Check sheet for the drawn part. Datum: minimum x, y, z corner. Units: mm. Give positions to 0.01 mm unless a question says otherwise; leave off trailing zeros. Order: outer loops, then holes, each group sorted by start corner. A loop starts at its lowest first (then second) coordinate and runs counter-clockwise, first axis right, second up. Notation, with made-up numbers: M 60.25,25.5 L 111.25,25.5 A32 cw 111.25,58.5 Z; hole C 22.25,81.25 d11. An arc over 180 degrees is marked long. Answer as CSV lines item,"result". Start each with the question number.
Q1. Section check D-D, the plane x = 92.5. Record the boundary of the cut face in (y, z).
Q2. Section check C-C, the plane z = 2.6. Record the boundary of the cut face in (x, y), then the cut area to 3 significant figures.
Q3. Section check A-A, the plane x = 42. Record the boundary of the cut face in (y, z).
Q4. Thickness scan on line 1 (X direction, y = 4, z = 1.95); line 2 (X direction, y = 11.5, z = 2.45); line 3 (Y direction, x = 42, z = 2.25). Record the ranges inside material, lowest first.
Q5. Section check B-B, the plane y = 4. Record the boundary of the cut face in (x, z).
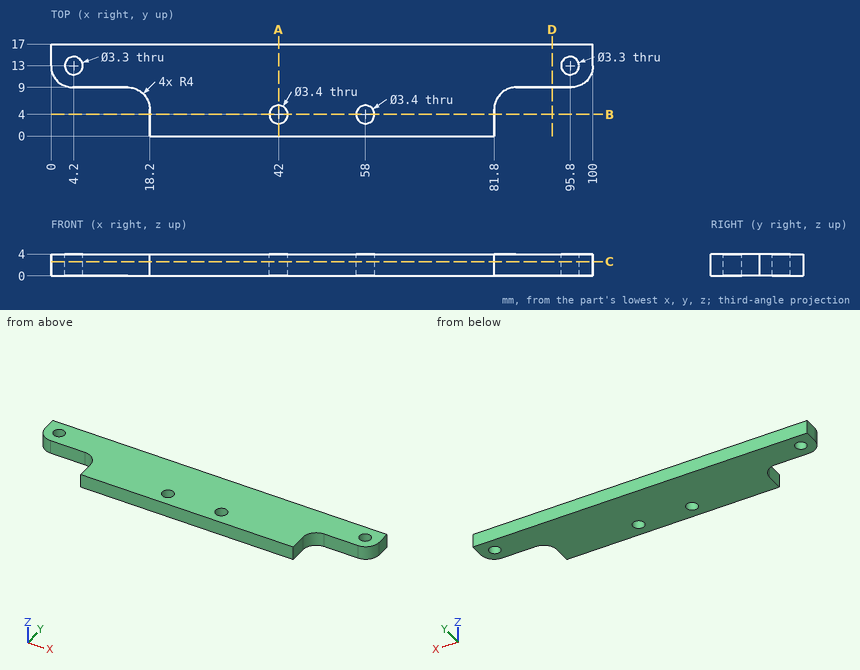
Answer block:
1,outline,"M 9,0 L 17,0 L 17,4 L 9,4 Z"
2,outline,"M 0,13 A4 ccw 4,9 L 14.2,9 A4 cw 18.2,5 L 18.2,0 L 81.8,0 L 81.8,5 A4 cw 85.8,9 L 96,9 A4 ccw 100,13 L 100,17 L 0,17 Z; hole C 4.2,13 d3.3; hole C 42,4 d3.4; hole C 58,4 d3.4; hole C 95.8,13 d3.3"
2,area,"1,340 mm2"
3,outline,"M 0,0 L 2.3,0 L 2.3,4 L 0,4 Z; M 5.7,0 L 17,0 L 17,4 L 5.7,4 Z"
4,line 1,"x = 18.2 to 40.3, 43.7 to 56.3, 59.7 to 81.8"
4,line 2,"x = 0.29 to 3.51, 4.89 to 95.11, 96.49 to 99.71"
4,line 3,"y = 0 to 2.3, 5.7 to 17"
5,outline,"M 18.2,0 L 40.3,0 L 40.3,4 L 18.2,4 Z; M 43.7,0 L 56.3,0 L 56.3,4 L 43.7,4 Z; M 59.7,0 L 81.8,0 L 81.8,4 L 59.7,4 Z"
